Model file for the job. Use its own axes, mm. Coordinates: 2 decimals unless noted, no trailing zeros. Order: outer loops, then holes, each group sorted by start corner. A loop starts at its lowest first (then second) coordinate and runs counter-clockwise, first axis right, second up. Notation, with made-up numbers: (-12.5, -2.5) -> (33.5, -2.5) arc R30 cw to (33.5, 32.5) -> close; hole circle Ø5 at (25.5, 5.5). An arc over 180 degrees is marked (long way). Write item = value, one per line. Start each with the question number.
Q1. Cut at B-B, the plane y = 13.5. List the corners of the cut face in (x, z), plus the area to 3 significant figures.
Q2. Wall check: line 1 (Y direction, x = 11.5, z = 0.2); line 2 (X direction, y = 15, z = 0.1); line 3 (Y direction, x = 10.75, z = 0.35). Give the ranges that are in metal, low to high. Write a range as from..to.
Q3. Cut at A-A, the plane y = 4.25. Give the number of separate pieces and of enclosed holes in the cut face, plus the area to 3 significant figures.
from build123d import *

# Parameters (mm, degrees)
SKETCH_1_R      = 0.499999
EXTRUDE_1_DEPTH = 0.41148


with BuildPart() as part:
    # 草图1 → 凸台-拉伸1 (new body)
    with BuildSketch(Plane(origin=(0, 0, 0), x_dir=(-1, 0, 0), z_dir=(0, 0, -1))):
        Polygon((-4.14330134, 3.23095112), (-4.02893784, 3.60795316), (-3.99032476, 3.99999962), (-4.00003264, 3.99999962), (-4.00003264, 20.00000064), (-3.99032222, 20.00000064), (-4.02893784, 20.39206742), (-4.1432988, 20.76906946), (-4.32901344, 21.11651606), (-4.57894436, 21.42105444), (-4.88348274, 21.67098536), (-5.23092934, 21.8567), (-5.60793138, 21.97106096), (-6.0000007, 22.00967658), (-6.0000007, 21.99997632), (-22.00000172, 21.99997632), (-22.00000172, 22.00967404), (-22.39207104, 21.97105842), (-22.76907054, 21.85669746), (-23.11651714, 21.67098282), (-23.42105806, 21.42105444), (-23.67098644, 21.11651352), (-23.85670108, 20.76906692), (-23.97106204, 20.39206742), (-24.00967766, 20.00000064), (-23.99999264, 20.00000064), (-23.99999264, 3.99999962), (-24.00967512, 3.99999962), (-23.9710595, 3.6079303), (-23.85669854, 3.2309308), (-23.6709839, 2.8834842), (-23.42105552, 2.57894328), (-23.1165146, 2.3290149), (-22.769068, 2.14330026), (-22.3920685, 2.0289393), (-22.00000172, 1.99032368), (-22.00000172, 2.00001632), (-5.999983914, 1.990341433), (-5.60793646, 2.02895454), (-5.23093442, 2.14331804), (-4.88348528, 2.32903268), (-4.57894436, 2.57896106), (-4.32901598, 2.88350198), align=None)
        with Locations(Location((-19.08001264, 19.74999352, 0), (0, 0, 180))):
            Circle(SKETCH_1_R, mode=Mode.SUBTRACT)
        with Locations(Location((-16.54001264, 19.74999352, 0), (0, 0, 180))):
            Circle(SKETCH_1_R, mode=Mode.SUBTRACT)
        with Locations(Location((-21.62001264, 19.74999352, 0), (0, 0, 180))):
            Circle(SKETCH_1_R, mode=Mode.SUBTRACT)
        with Locations(Location((-11.46001264, 19.74999352, 0), (0, 0, 180))):
            Circle(SKETCH_1_R, mode=Mode.SUBTRACT)
        with Locations(Location((-14.00001264, 19.74999352, 0), (0, 0, 180))):
            Circle(SKETCH_1_R, mode=Mode.SUBTRACT)
        with Locations(Location((-19.08001264, 4.24999912, 0), (0, 0, 180))):
            Circle(SKETCH_1_R, mode=Mode.SUBTRACT)
        with Locations(Location((-21.62001264, 4.24999912, 0), (0, 0, 180))):
            Circle(SKETCH_1_R, mode=Mode.SUBTRACT)
        with Locations(Location((-14.00001264, 4.24999912, 0), (0, 0, 180))):
            Circle(SKETCH_1_R, mode=Mode.SUBTRACT)
        with Locations(Location((-16.54001264, 4.24999912, 0), (0, 0, 180))):
            Circle(SKETCH_1_R, mode=Mode.SUBTRACT)
        with Locations(Location((-8.92001264, 19.74999352, 0), (0, 0, 180))):
            Circle(SKETCH_1_R, mode=Mode.SUBTRACT)
        with Locations(Location((-6.38001264, 19.74999352, 0), (0, 0, 180))):
            Circle(SKETCH_1_R, mode=Mode.SUBTRACT)
        with Locations(Location((-6.00002864, 15.80999632, 0), (0, 0, 180))):
            Circle(SKETCH_1_R, mode=Mode.SUBTRACT)
        with Locations(Location((-6.00002864, 13.26999632, 0), (0, 0, 180))):
            Circle(SKETCH_1_R, mode=Mode.SUBTRACT)
        with Locations(Location((-6.00002864, 10.72999632, 0), (0, 0, 180))):
            Circle(SKETCH_1_R, mode=Mode.SUBTRACT)
        with Locations(Location((-8.92001264, 4.24999912, 0), (0, 0, 180))):
            Circle(SKETCH_1_R, mode=Mode.SUBTRACT)
        with Locations(Location((-11.46001264, 4.24999912, 0), (0, 0, 180))):
            Circle(SKETCH_1_R, mode=Mode.SUBTRACT)
        with Locations(Location((-6.00002864, 8.18999632, 0), (0, 0, 180))):
            Circle(SKETCH_1_R, mode=Mode.SUBTRACT)
        with Locations(Location((-6.38001264, 4.24999912, 0), (0, 0, 180))):
            Circle(SKETCH_1_R, mode=Mode.SUBTRACT)
    extrude(amount=-EXTRUDE_1_DEPTH)


solid = part.part
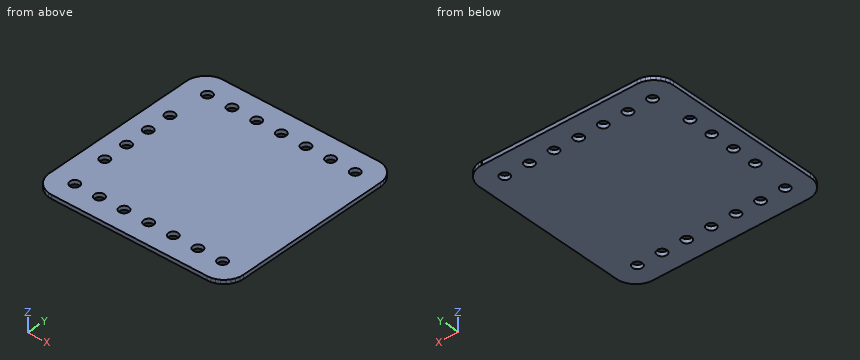
Here are the results:
q1.outline = (4, 0) -> (5.56, 0) -> (5.56, 0.41) -> (4, 0.41) -> close; (6.44, 0) -> (24, 0) -> (24, 0.41) -> (6.44, 0.41) -> close
q1.area = 7.86 mm²
q2.line_1 = 1.99..3.75, 4.75..19.25, 20.25..22
q2.line_2 = 4..24
q2.line_3 = 1.99..22
q3.separate_pieces = 8
q3.enclosed_holes = 0
q3.area = 5.35 mm²
